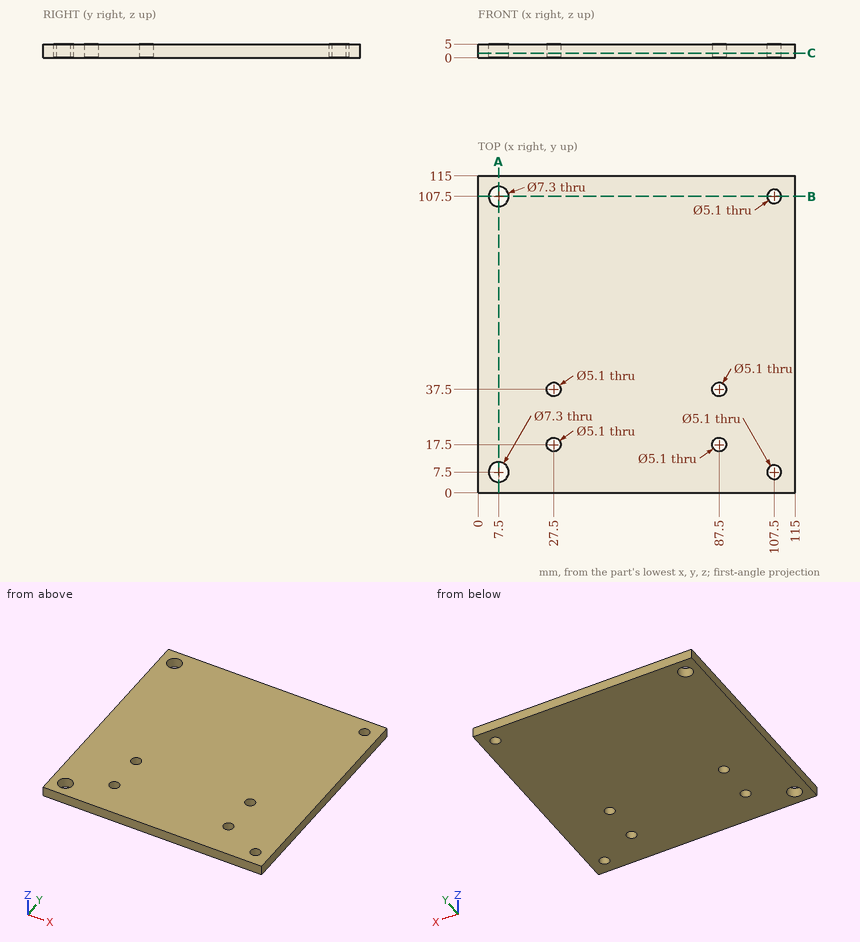
Design review of the part shown in the three views and the two pictorial views. Dimensions are in mm from the part's minimum x, y and z. Coordinates: 2 decimals unless noted, no trailing zeros. Loops run counter-clockwise (first coordinate to the right, second up) from the corner with the lowest first, then second, coordinate; pieces in that order, holes last.
(1) Consider section B-B, the plane y = 107.5. Give the boundary of the cut face in (x, z).
Determined:
outline: (0, 0) - (3.85, 0) - (3.85, 5) - (0, 5) - close; (11.15, 0) - (104.95, 0) - (104.95, 5) - (11.15, 5) - close; (110.05, 0) - (115, 0) - (115, 5) - (110.05, 5) - close
(2) Consider section A-A, the plane x = 7.5. Give the boundary of the cut face in (y, z).
Determined:
outline: (0, 0) - (3.85, 0) - (3.85, 5) - (0, 5) - close; (11.15, 0) - (103.85, 0) - (103.85, 5) - (11.15, 5) - close; (111.15, 0) - (115, 0) - (115, 5) - (111.15, 5) - close
(3) Consider section C-C, the plane z = 1.65. Give the number of separate pieces and of enclosed holes in the cut face, plus the area to 3 significant figures.
Determined:
separate pieces: 1
enclosed holes: 8
area: 13,000 mm2
(4) Wall thickness on L1, parallel to Y at x = 107.5, z = 3.8; L2, parallel to X at y = 7.5, z = 1.75; L3, parallel to Y at x = 7.5, z = 2.05: over which ranges is each line inside the solid? List them lowest first.
Determined:
L1: y = 0 to 4.95, 10.05 to 104.95, 110.05 to 115
L2: x = 0 to 3.85, 11.15 to 104.95, 110.05 to 115
L3: y = 0 to 3.85, 11.15 to 103.85, 111.15 to 115
